Geometry check sheet. Reference: the model listing, model coordinates, mm. Round coordinates to 2 decimals unless told otherwise and drop trailing zeros. Order: outer loops, then holes, each group sorted by start corner. A loop starts at its lowest first (then second) coordinate and runs counter-clockwise, first axis right, second up. Notation, with made-up numbers: (61.25, -10.5) - (73.25, -10.5) arc R19 ccw to (73.25, -4.5) - close; hole circle Ø1 at (15, 72.25). An arc over 180 degrees is marked (long way). One line per question, with ' | ' between items. Start each with the question number.
Q1. Sectioned sample at B-B, the plane x = 12.25. Enter the section's corners in (y, z).
Q2. Sectioned sample at A-A, the plane y = -5.1. Enter the section's corners in (x, z), then the cut area to 3 significant figures.
Q3. Gauge pin test, flat ends, axial feed: P1, Ø1, axis at x = 11, z = 4, coming from the +Y side; P2, Ø1, axis at x = 11, z = 1.5, coming from the -Y side; P3, Ø1, axis at x = 11.5, z = 2.5, coming from the -Y side. Record the tip position at first contact, or that the pin passes through.
Q4. Material ranges on line 1 along Y through (x, z) = (13.1, 4.25); line 2 along X through (y, z) = (-5.3, 4.5); line 3 along Y through (x, z) = (12.8, 4.5), recorded low to high.
Q5. Sectioned sample at C-C, the plane z = 1.25. Enter the section's corners in (x, y).
Autodesk Inventor part; units mm, degrees
ref_plane "YZ Plane" through (0, 0, 0) normal (1, 0, 0) x (0, 1, 0)
ref_plane "XZ Plane" through (0, 0, 0) normal (0, 1, 0) x (-1, 0, 0)
ref_plane "XY Plane" through (0, 0, 0) normal (0, 0, 1) x (1, 0, 0)
sketch "Sketch1" plane through (0, 0, 0) normal (0, 0, 1) x (1, 0, 0)
  arc A0 (13.554, -7.5586) -> (10.818, -7.5586) centre (12.186, -6.0655) ccw
  arc A1 (12.5997, -7.5323) -> (11.7723, -7.5323) centre (12.186, -6.0655) ccw
  arc A2 (13.5197, -7.5211) -> (10.8523, -7.5211) centre (12.186, -6.0655) ccw
  arc A3 (12.6342, -7.6545) -> (11.7378, -7.6545) centre (12.186, -6.0655) ccw
  circle A4 centre (12.186, -6.0655) radius 1.651
  circle A5 centre (12.186, -6.0655) radius 1.9742
  point P0 (0, 0)
  dimension "d0" = 0.0508
  dimension "d1" = 0.127
extrude "Extrusion1" add sketch "Sketch1" along normal blind 6.9342
properties part number "ServoSpacer"
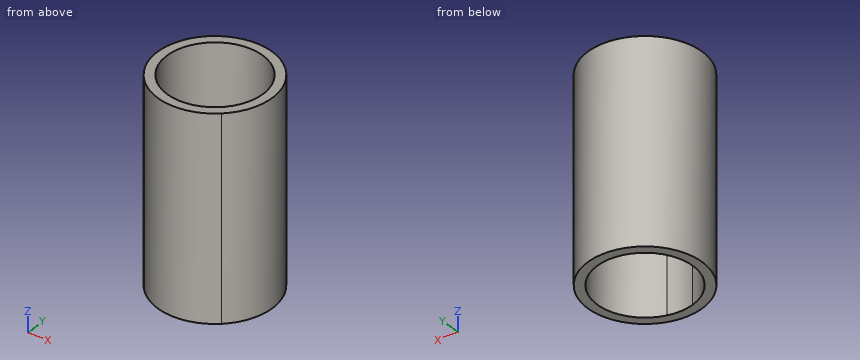
Determined:
1) outline: (-8.04, 0) - (-7.72, 0) - (-7.72, 6.93) - (-8.04, 6.93) - close; (-4.42, 0) - (-4.09, 0) - (-4.09, 6.93) - (-4.42, 6.93) - close
2) outline: (10.46, 0) - (10.85, 0) - (10.85, 6.93) - (10.46, 6.93) - close; (13.53, 0) - (13.91, 0) - (13.91, 6.93) - (13.53, 6.93) - close | area: 5.31 mm2
3) P1: stops at y = -4.21 | P2: stops at y = -7.92 | P3: stops at y = -8.03
4) line 1: y = -7.82 to -7.44, -4.69 to -4.32 | line 2: x = 10.37 to 10.72, 13.65 to 14.01 | line 3: y = -7.94 to -7.6, -4.53 to -4.19
5) outline: circle Ø3.95 at (12.19, -6.07); hole circle Ø3.3 at (12.19, -6.07)
